from build123d import *

# Parameters (mm, degrees)
SKETCH1_R           = 10.5
SKETCH1_R_2         = 8
BOSS_EXTRUDE1_DEPTH = 0.4
SKETCH2_R           = 0.75
BOSS_EXTRUDE2_DEPTH = 1
SKETCH3_R           = 0.5
BOSS_EXTRUDE3_DEPTH = 1
CIRPATTERN1_COUNT   = 4
DRAFT1_ANGLE        = 1


with BuildPart() as part:
    # Sketch1 → Boss-Extrude1 (new body)
    with BuildSketch(Plane(origin=(0, 0, 0), x_dir=(1, 0, 0), z_dir=(0, 1, 0))):
        with Locations(Location((0, 1.53064501, 0), (0, 0, 270))):
            Circle(SKETCH1_R)
        with Locations(Location((0, 1.53064501, 0), (0, 0, 270))):
            Circle(SKETCH1_R_2, mode=Mode.SUBTRACT)
    extrude(amount=BOSS_EXTRUDE1_DEPTH)

    # Sketch2 → Boss-Extrude2 (add)
    with BuildSketch(Plane(origin=(0, 0, 0), x_dir=(1, 0, 0), z_dir=(0, 1, 0))):
        with Locations(Location((-6.717514421, -5.186869411, 0), (0, 0, 270))):
            Circle(SKETCH2_R)
    boss_extrude2 = extrude(amount=-BOSS_EXTRUDE2_DEPTH)

    # Sketch3 → Boss-Extrude3 (add)
    with BuildSketch(Plane.XZ.offset(1)):
        with Locations(Location((-6.717514421, 5.186869411, 0), (0, 0, 270))):
            Circle(SKETCH3_R)
    boss_extrude3 = extrude(amount=BOSS_EXTRUDE3_DEPTH)

    # CirPattern1: Boss-Extrude2, Boss-Extrude3 ×4 about axis
    cirpattern1_axis = Axis((0, 0, -1.53064501), (0, 1, 0))
    add([boss_extrude2.rotate(cirpattern1_axis, i * 360 / CIRPATTERN1_COUNT) for i in range(1, CIRPATTERN1_COUNT)])
    add([boss_extrude3.rotate(cirpattern1_axis, i * 360 / CIRPATTERN1_COUNT) for i in range(1, CIRPATTERN1_COUNT)])

    # Draft1
    draft1_faces = [part.faces().sort_by_distance(p)[0] for p in [
        (5.967514421, -0.5, 5.186869411),
        (7.217514421, -1.5, 5.186869411),
        (6.717514421, -0.5, -7.498159431),
        (6.717514421, -1.5, -8.748159431),
        (-5.967514421, -0.5, -8.248159431),
        (-7.217514421, -1.5, -8.248159431),
        (-6.717514421, -0.5, 4.436869411),
        (-6.717514421, -1.5, 5.686869411),
    ]]
    draft(draft1_faces, Plane(origin=(0, 0, -1.53064501), x_dir=(0, 0, -1), z_dir=(0, -1, 0)), DRAFT1_ANGLE)


solid = part.part
Part model, mm, in its own coordinate system. A direction names the side the tool comes from. Give positions to 0.01 mm unless a question says otherwise; leave off trailing zeros. Loops run counter-clockwise (first coordinate to the right, second up) from the corner with the lowest first, then second, coordinate; pieces in that order, holes last. Notation, with made-up numbers: (21.25, 9.5) -> (27.25, 9.5) arc R23 cw to (27.25, 26.5) -> close; hole circle Ø7 at (61.5, -6.75). An arc over 180 degrees is marked (long way). Write each question's results on one line, items separated by ' | '. Start each with the question number.
Q1. Pin check, flat tips, straight feed: P1, Ø1, axis at y = 0, z = -7.5, coming from the +X side; P2, Ø1.5, axis at x = -6, z = -4.5, coming from the +Y side. Stop position of each tip, or through.
Q2. Pull direction Z, two halves, no side cores. Call faces 1 (the face through (-8, 0.4, -4)), 2 (the face through (3.154, 0.197, 8.484)), 3 (the face through (-7.001, -0.493, 5.872)): +Z half, -Z half, draft (parallel to the pull), parting line (faces both ways), or undercut.
Q3. Which spindle directions (+Z, -Z, +X, -X, +Y, -Y) get a long thin tool onto all of the face, cutting with end or side? Do faces 4 (the face through (7.425, -0.493, 4.964)), 5 (the face through (-7.8, 0.2, -3.3)). Say none if no direction does.
Q4. Band-saw the part on A-A on x = 0. List the corners of the cut face in (y, z).
Q5. Band-saw the part on C-C on y = -1.65. List the corners of the cut face in (x, z), plus the area to 3 significant figures.
Q6. Band-saw the part on B-B on z = -1.5. List the corners of the cut face in (x, y), plus the area to 3 significant figures.
Q7. Wall check: L1, parallel to Y at x = -9.5, z = -4; L2, parallel to X at y = 0.05, z = 1.5; L3, parallel to Z at x = -7, y = -1.8. Give the ranges that are in metal, low to high.
Results are:
1) P1: stops at x = 8.96 | P2: passes through
2) face 1: draft | face 2: parting line | face 3: undercut
3) face 4: -Y | face 5: +Y, -Y
4) outline: (0, -12.03) -> (0.4, -12.03) -> (0.4, -9.53) -> (0, -9.53) -> close; (0, 6.47) -> (0.4, 6.47) -> (0.4, 8.97) -> (0, 8.97) -> close
5) outline: circle Ø0.94 at (-6.72, -8.25); circle Ø0.94 at (-6.72, 5.19); circle Ø0.94 at (6.72, -8.25); circle Ø0.94 at (6.72, 5.19) | area: 2.79 mm²
6) outline: (-10.5, 0) -> (-8, 0) -> (-8, 0.4) -> (-10.5, 0.4) -> close; (8, 0) -> (10.5, 0) -> (10.5, 0.4) -> (8, 0.4) -> close | area: 2.00 mm²
7) L1: y = 0 to 0.4 | L2: x = -10.05 to -7.4, 7.4 to 10.05 | L3: z = -8.62 to -7.87, 4.81 to 5.56
